Build history of the part. All positions in model axes, mm. A direction names the side the tool comes from. Round coordinates to 2 decimals unless told otherwise and drop trailing zeros. Loops run counter-clockwise (first coordinate to the right, second up) from the corner with the lowest first, then second, coordinate; pieces in that order, holes last. Notation, with made-up numbers: M -20.75,-21.5 L 2.25,-21.5 A15 cw 2.25,-3.5 Z; hole C 54,58.25 d7. An arc over 180 degrees is marked long. One line per item, written item: value.
```python
from build123d import *

# Parameters (mm, degrees)
F3_D           = 14.2875
F4_D           = 8.4074
F4_CSINK_D     = 10.922
F4_CSINK_ANGLE = 90
F5_D           = 4.3688
F5_CSINK_D     = 8.128
F5_CSINK_ANGLE = 82
F6_SIZE2       = 0.254
F6_SIZE        = 0.254


with BuildPart() as f1:
    # F0 (on Right) → F1 (revolve)
    with BuildSketch(Plane.YZ):
        Polygon((4.7498, 24.4475), (0, 24.4475), (0, 0), (9.4996, 0), (9.4996, 25.4), (4.7498, 25.4), align=None)
    revolve(axis=Axis((0, 5.1186173223, 0), (0, 1, 0)))

    # F3 (through all)
    with Locations(Plane(origin=(0, 9.4996, 0), x_dir=(-1, 0, 0), z_dir=(0, 1, 0))):
        with Locations((0, -14.732)):
            Hole(F3_D / 2)

    # F4 (through all)
    with Locations(Plane(origin=(0, 9.4996, 0), x_dir=(-1, 0, 0), z_dir=(0, 1, 0))):
        with Locations((0, 14.732)):
            CounterSinkHole(F4_D / 2, F4_CSINK_D / 2, counter_sink_angle=F4_CSINK_ANGLE)

    # F5 (through all)
    with Locations(Plane(origin=(0, 9.4996, 0), x_dir=(-1, 0, 0), z_dir=(0, 1, 0))):
        with Locations((-17.78, 0), (17.78, 0)):
            CounterSinkHole(F5_D / 2, F5_CSINK_D / 2, counter_sink_angle=F5_CSINK_ANGLE)

    # F6
    f6_edges = [f1.edges().sort_by_distance(p)[0] for p in [
        (0, 9.4996, -25.4),
        (0, 0, -24.4475),
        (0, 4.7498, -25.4),
        (7.14375, 0, -14.732),
        (4.2037, 0, 14.732),
        (7.14375, 9.4996, -14.732),
    ]]
    chamfer(f6_edges, length=F6_SIZE, length2=F6_SIZE2)


solid = f1.part
```
Item 1: Slice it at C-C, the plane y = 6.75. Give the cut face in (x, z), and give its area (3 significant figures).
Check values:
outline: C 0,0 d50.8; hole C -17.78,0 d4.37; hole C 0,-14.73 d14.29; hole C 0,14.73 d8.41; hole C 17.78,0 d4.37
area: 1,780 mm2
Item 2: Drop flat-ended pins along their axis: P1, Ø7.5, axis at x = 0, z = 14.732, coming from the +Y side; P2, Ø1.5, axis at y = 5.5, z = -6.5, coming from the -X side; P3, Ø1, axis at x = 9, y = 5, coming from the +Z side; P4, Ø1.5, axis at x = 16.5, y = 6.5, coming from the +Z side. Give the stop position or say it passes through.
Check values:
P1: passes through
P2: stops at x = -24.74
P3: stops at z = 23.94
P4: stops at z = 19.93
Item 3: Wall check: line 1 along X through (y, z) = (2.5, 0); line 2 along X through (y, z) = (6.5, -2); line 3 along Z through (x, y) = (-1.5, 7.5). Give the ranges that are in metal, low to high.
Check values:
line 1: x = -24.45 to -19.96, -15.6 to 15.6, 19.96 to 24.45
line 2: x = -25.32 to -18.66, -16.9 to 16.9, 18.66 to 25.32
line 3: z = -25.36 to -21.72, -7.75 to 10.81, 18.66 to 25.36
Item 4: Which spindle directions (+Z, -Z, +X, -X, +Y, -Y) get a long thin tool onto all of the face, cutting with end or side? Do faces 4 (the face through (-23.866, 2.47, -5.3)), 5 (the face through (0, 0, 0)). Say none if no direction does.
Check values:
face 4: -Y
face 5: +Z, -Z, +X, -X, -Y
Item 5: Slice it at B-B, the plane z = 0. Give the cut face in (x, y), and give its area (3 significant figures).
Check values:
outline: M -25.4,5 L -25.15,4.75 L -24.45,4.75 L -24.45,0.25 L -24.19,0 L -19.96,0 L -19.96,7.34 L -21.84,9.5 L -25.15,9.5 L -25.4,9.25 Z; M -15.6,0 L 15.6,0 L 15.6,7.34 L 13.72,9.5 L -13.72,9.5 L -15.6,7.34 Z; M 19.96,0 L 24.19,0 L 24.45,0.25 L 24.45,4.75 L 25.15,4.75 L 25.4,5 L 25.4,9.25 L 25.15,9.5 L 21.84,9.5 L 19.96,7.34 Z
area: 382 mm2
Item 6: Slice it at A-A, the plane x = 0. Give the number of separate pieces and of enclosed holes in the cut face, and give its area (3 significant figures).
Check values:
separate pieces: 3
enclosed holes: 0
area: 256 mm2
Item 7: Pull direction X, two halves, no side cores. Call faces 1 (the face through (-24.796, 7.095, -5.506)), 2 (the face through (-15.762, 3.617, -0.837)), 3 (the face through (0, 9.5, 0)): pulls with the +X half, pulls with the -X half, needs draft (parallel to the pull), parting line crosses it, or undercut.
Check values:
face 1: parting line crosses it
face 2: undercut
face 3: needs draft
